```python
from build123d import *

# Parameters (mm, degrees)
F1_DEPTH = 6.35


# Not quite as in the source:
# - a feature names something its author has since deleted; it is built from what else it names


with BuildPart() as f1:
    # F0 (on Top) → F1 (new body)
    with BuildSketch(Plane.XY):
        Polygon((44.45, 19.05), (38.1, 19.05), (-38.1, 19.05), (-44.45, 19.05), (-44.45, 6.35), (-38.1, 6.35), (-38.1, -6.35), (-44.45, -6.35), (-44.45, -19.05), (-38.1, -19.05), (38.1, -19.05), (44.45, -19.05), (44.45, -6.35), (38.1, -6.35), (38.1, 6.35), (44.45, 6.35), align=None)
    extrude(amount=F1_DEPTH)


solid = f1.part
```
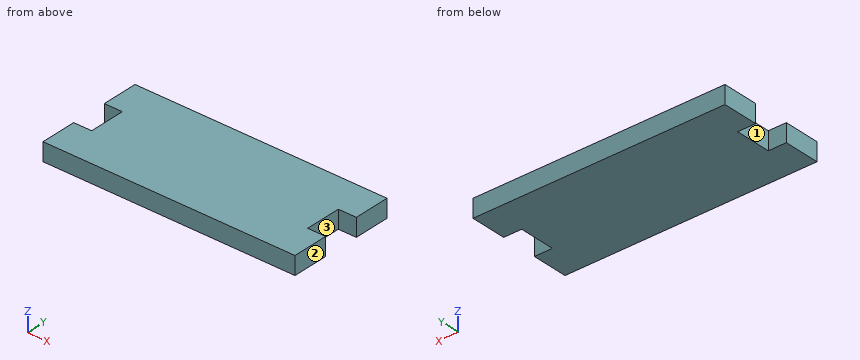
Here's how the part is built. I have some questions about the finished solid (model axes, mm). Face numbers are marked on the shaded views. A direction names the side the tool comes from. Round coordinates to 2 decimals unless told otherwise and drop trailing zeros. Write each loop counter-clockwise with the first axis right and the second up, starting at its lowest first coordinate (ties: lowest second). Pieces come first, ordered by that corner, then holes.
Q1. If we section it at A-A on z = 3.5: Write out the boundary of the cut face in (x, y), plus the area to 3 significant figures.
Q2. If we section it at B-B on y = -3: Write out the boundary of the cut face in (x, z).
Q3. Will this pin go through, and if not, where does the flat tip stop? P1, Ø3, axis at y = 2, z = 4.5, coming from the -X side.
Q4. Please list where this line runs through material, in increasing order: probe 1 along X at (y, z) = (0, 2.5).
Q5. Which directions (+Z, -Z, +X, -X, +Y, -Y) give clear straight access to the entire face, cutting with the end or side of a thin tool? Please do the marked faces 1, 2 and 3.
Answer below:
1. outline: (-44.45, -19.05) - (44.45, -19.05) - (44.45, -6.35) - (38.1, -6.35) - (38.1, 6.35) - (44.45, 6.35) - (44.45, 19.05) - (-44.45, 19.05) - (-44.45, 6.35) - (-38.1, 6.35) - (-38.1, -6.35) - (-44.45, -6.35) - close
1. area: 3,230 mm2
2. outline: (-38.1, 0) - (38.1, 0) - (38.1, 6.35) - (-38.1, 6.35) - close
3. P1: stops at x = -38.1
4. probe 1: x = -38.1 to 38.1
5. face 1: +Z, -Z, -X
5. face 2: +Z, -Z, +X, +Y, -Y
5. face 3: +Z, -Z, +X
